from build123d import *

# Parameters (mm, degrees)
SKETCH1_R           = 3
BOSS_EXTRUDE1_DEPTH = 5


with BuildPart() as part:
    # Sketch1 → Boss-Extrude1 (new body)
    with BuildSketch(Plane(origin=(0, 0, 0), x_dir=(1, 0, 0), z_dir=(0, 1, 0))):
        with BuildLine():
            Line((0, 7.5), (20, 7.5))
            ThreePointArc((20, 7.5), (27.5, 0), (20, -7.5))
            Line((20, -7.5), (0, -7.5))
            ThreePointArc((0, -7.5), (-7.5, 0), (0, 7.5))
        make_face()
        with Locations(Location((20, 0, 0), (0, 0, 270))):
            Circle(SKETCH1_R, mode=Mode.SUBTRACT)
        with BuildLine():
            Line((1.5, 2), (-1.5, 2))
            ThreePointArc((-1.5, 2), (0, -2.5), (1.5, 2))
        make_face(mode=Mode.SUBTRACT)
    extrude(amount=BOSS_EXTRUDE1_DEPTH)


solid = part.part
Read the model definition and answer for the solid it produces. Units are mm, in the model's axes. Coordinates: 2 decimals unless noted, no trailing zeros. Order: outer loops, then holes, each group sorted by start corner. A loop starts at its lowest first (then second) coordinate and runs counter-clockwise, first axis right, second up. Notation, with made-up numbers: (44, -21) -> (50, -21) arc R21 ccw to (50, -9) -> close; hole circle Ø3 at (61.5, 3). An arc over 180 degrees is marked (long way). Answer as a JSON object with one key per item and string values.
1) Consider line 1 along X through (y, z) = (1.45, 0); line 2 along Z through (x, y) = (0, 2.2); line 3 along X through (y, z) = (0.75, 2.75). Determine where each line is inside the solid, lowest interval first. Write a range as from..to.
Model answer:
{"line 1": "x = -7.5..-2.5, 2.5..17, 23..27.5", "line 2": "z = -7.5..-2, 2.5..7.5", "line 3": "x = -6.98..18.8, 21.2..26.98"}
2) A cutting plane is placed at B-B, the plane y = 0.95. Determine the outline of the cut face in (x, z).
Model answer:
{"outline": "(0, -7.5) -> (20, -7.5) arc R7.5 ccw to (20, 7.5) -> (0, 7.5) arc R7.5 ccw to start; hole (-1.5, -2) -> (1.5, -2) arc R2.5 ccw (long way) to start; hole circle Ø6 at (20, 0)"}
3) A cutting plane is placed at A-A, the plane z = 0. Determine the outline of the cut face in (x, y), plus the area to 3 significant figures.
Model answer:
{"outline": "(-7.5, 0) -> (-2.5, 0) -> (-2.5, 5) -> (-7.5, 5) -> close; (2.5, 0) -> (17, 0) -> (17, 5) -> (2.5, 5) -> close; (23, 0) -> (27.5, 0) -> (27.5, 5) -> (23, 5) -> close", "area": "120 mm²"}
4) Each of these flat-tipped pins is pushed along its axis until it touches: pin 1 (1.5 mm diameter, centred on x = 21.5, z = 0.5, fed in from +Y); pin 2 (3 mm diameter, centred on y = 2.5, z = 6, fed in from +X); pin 3 (2 mm diameter, centred on y = 3, z = -2.5, fed in from -X); pin 4 (2 mm diameter, centred on y = 4.5, z = 2, fed in from -X). Where does it stop, or does it pass through?
Model answer:
{"pin 1": "passes through", "pin 2": "stops at x = 26", "pin 3": "stops at x = -7.35", "pin 4": "stops at x = -7.43"}
5) A cutting plane is placed at D-D, the plane z = 5. Determine the outline of the cut face in (x, y).
Model answer:
{"outline": "(-5.59, 0) -> (25.59, 0) -> (25.59, 5) -> (-5.59, 5) -> close"}
6) A cutting plane is placed at C-C, the plane x = 24.5. Determine the outline of the cut face in (y, z), plus the area to 3 significant figures.
Model answer:
{"outline": "(0, -6) -> (5, -6) -> (5, 6) -> (0, 6) -> close", "area": "60.0 mm²"}
7) The mould has two halves that part along X. Classify faces 1 (the face through (17.07, 2.46, -0.65)), 2 (the face through (0, 2, -2)), 3 (the face through (10, 2, 7.5)), 4 (the face through (27.5, 2.46, -0.16)): released by +X, released by -X, zero draft, split by the parting line, or undercut.
Model answer:
{"face 1": "undercut", "face 2": "undercut", "face 3": "zero draft", "face 4": "released by +X"}
